Can you work these out from the drawing? Everything is in mm from the part's minimum corner. A direction names the side the tool comes from. Round coordinates to 2 decimals unless told otherwise and drop trailing zeros. Loops run counter-clockwise (first coordinate to the right, second up) from the corner with the lowest first, then second, coordinate; pieces in that order, holes last. Notation, with made-up numbers: (-15.75, 75) -> (-9.75, 75) arc R22 cw to (-9.75, 83) -> close; hole circle Ø11 at (12, 72). An arc over 180 degrees is marked (long way). One line per item, written item: value.
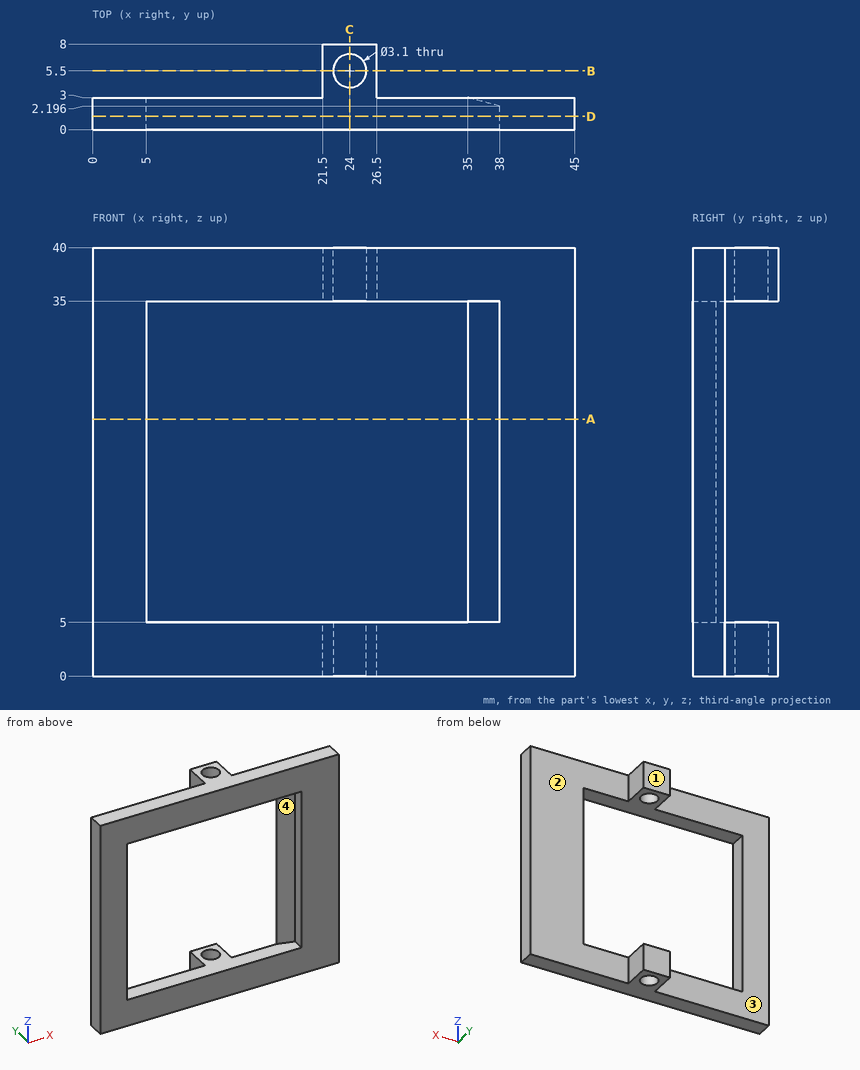
Item 1: Will these pins go through, and if not, where does the flat tip stop? pin 1 Ø2.5 at (y, z) = (6, 2.5) entering from +X; pin 2 Ø12 at (x, z) = (7, 6.5) entering from -Y; pin 3 Ø1 at (x, z) = (37, 5) entering from +Y; pin 4 Ø2.5 at (y, z) = (5, 3) entering from -X.
Output:
pin 1: stops at x = 26.5
pin 2: stops at y = 0
pin 3: stops at y = 3
pin 4: stops at x = 21.5
Item 2: For the marked faces 1 and 2, which set-ups out of +Z, -Z, +X, -X, +Y, -Y let a thin tool reach every point of the face, with its end or its side?
Output:
face 1: +Z, -Z, +X, -X, +Y
face 2: +Z, -Z, +X, +Y
Item 3: If we section it at A-A on z = 24: List the corners of the cut face in (x, y) for me.
Output:
outline: (0, 0) -> (5, 0) -> (5, 3) -> (0, 3) -> close; (35, 3) -> (38, 2.2) -> (38, 0) -> (45, 0) -> (45, 3) -> close
Item 4: If we section it at C-C on x = 24: List the corners of the cut face in (y, z) for me, plus the area to 3 significant figures.
Output:
outline: (0, 0) -> (3.95, 0) -> (3.95, 5) -> (0, 5) -> close; (0, 35) -> (3.95, 35) -> (3.95, 40) -> (0, 40) -> close; (7.05, 0) -> (8, 0) -> (8, 5) -> (7.05, 5) -> close; (7.05, 35) -> (8, 35) -> (8, 40) -> (7.05, 40) -> close
area: 49.0 mm²
Item 5: I need wall thicknesses on line 1 (Z direction, x = 17.5, y = 2.5); line 2 (Y direction, x = 42.5, z = 19.5); line 3 (Y direction, x = 25, z = 37) (1 decimal). Which ranges of each line are inside material? Lowest first, please. Write a range as from..to.
Output:
line 1: z = 0..5, 35..40
line 2: y = 0..3
line 3: y = 0..4.3, 6.7..8
Item 6: If we mould it in two halves opening along Z, with no side actions, what happens to the marked faces 3 and 4? For each: released by +Z, released by -Z, zero draft, split by the parting line, or undercut.
Output:
face 3: zero draft
face 4: undercut
Item 7: If we section it at D-D on y = 1.25: List the corners of the cut face in (x, z) for me.
Output:
outline: (0, 0) -> (45, 0) -> (45, 40) -> (0, 40) -> close; hole (5, 5) -> (38, 5) -> (38, 35) -> (5, 35) -> close
Item 8: If we section it at B-B on y = 5.5: List the corners of the cut face in (x, z) for me, plus the area to 3 significant figures.
Output:
outline: (21.5, 0) -> (22.45, 0) -> (22.45, 5) -> (21.5, 5) -> close; (21.5, 35) -> (22.45, 35) -> (22.45, 40) -> (21.5, 40) -> close; (25.55, 0) -> (26.5, 0) -> (26.5, 5) -> (25.55, 5) -> close; (25.55, 35) -> (26.5, 35) -> (26.5, 40) -> (25.55, 40) -> close
area: 19.0 mm²
